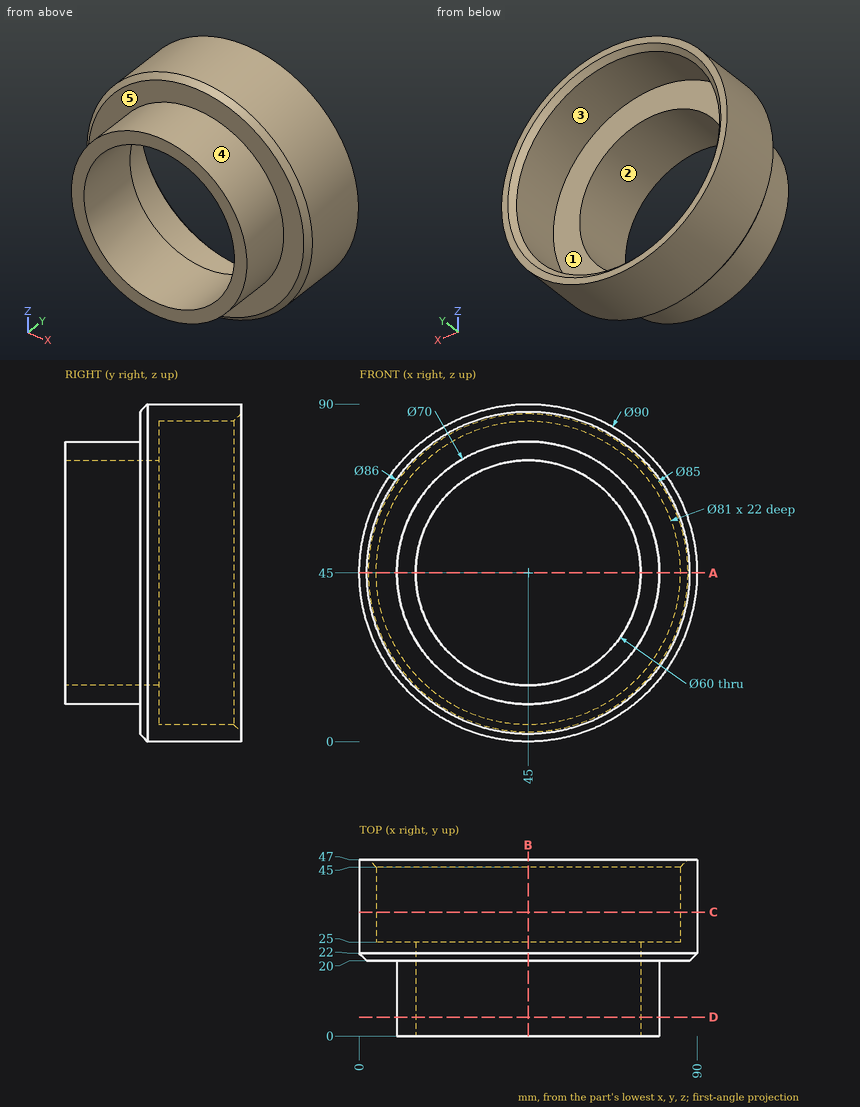
Could you check a few things on this drawing? It's one solid part, dimensions in mm from its lowest x, y, z. A direction names the side the tool comes from. Give positions to 0.01 mm unless a question says otherwise; leave off trailing zeros. Write each loop counter-clockwise with the first axis right and the second up, starting at its lowest first coordinate (ties: lowest second). Pieces come first, ordered by that corner, then holes.
(1) Imagine slicing it at A-A, the plane z = 45. Write out the boundary of the cut face in (x, y), and give its area (3 significant figures).
Output values:
outline: (0, 22) - (2, 20) - (10, 20) - (10, 0) - (15, 0) - (15, 25) - (4.5, 25) - (4.5, 45) - (2.5, 47) - (0, 47) - close; (75, 0) - (80, 0) - (80, 20) - (88, 20) - (90, 22) - (90, 47) - (87.5, 47) - (85.5, 45) - (85.5, 25) - (75, 25) - close
area: 540 mm2
(2) On a 3-axis mill with a long thin cutter (end or side, diameter ignored), from which of +Z, -Z, +X, -X, +Y, -Y can I reach the whole of each face in a straight line? I mean the marked faces 1 and 2. Say none if no direction works.
Output values:
face 1: +Y
face 2: +Y, -Y
(3) Imagine slicing it at D-D, the plane y = 5. Write out the boundary of the cut face in (x, z), and give its area (3 significant figures).
Output values:
outline: circle Ø70 at (45, 45); hole circle Ø60 at (45, 45)
area: 1,020 mm2
(4) If I drill on L1, parallel to X at y = 15.5, z = 45; L2, parallel to X at y = 35, z = 45, over which ranges is the centre line in solid material (lowest first)?
Output values:
L1: x = 10 to 15, 75 to 80
L2: x = 0 to 4.5, 85.5 to 90
(5) Will these pins go through, and if not, where does the flat tip stop? pin 1 (8 mm diameter, centred on y = 33.5, z = 65.5, fed in from -X); pin 2 (6 mm diameter, centred on x = 69.5, z = 26.5, fed in from +Y); pin 3 (1 mm diameter, centred on y = 5.5, z = 61, fed in from -X).
Output values:
pin 1: stops at x = 3.13
pin 2: stops at y = 25
pin 3: stops at x = 13.62
(6) Thinking about a two-plate mould opening in X: for the marked faces 3, 4 and 5, which applies, pulls with the +X half, pulls with the -X half, needs draft (parallel to the pull), parting line crosses it, or undercut?
Output values:
face 3: undercut
face 4: parting line crosses it
face 5: needs draft
(7) Imagine slicing it at B-B, the plane x = 45. Write out the boundary of the cut face in (y, z), and give its area (3 significant figures).
Output values:
outline: (0, 10) - (20, 10) - (20, 2) - (22, 0) - (47, 0) - (47, 2.5) - (45, 4.5) - (25, 4.5) - (25, 15) - (0, 15) - close; (0, 75) - (25, 75) - (25, 85.5) - (45, 85.5) - (47, 87.5) - (47, 90) - (22, 90) - (20, 88) - (20, 80) - (0, 80) - close
area: 540 mm2
(8) Imagine slicing it at C-C, the plane y = 33. Write out the boundary of the cut face in (x, z).
Output values:
outline: circle Ø90 at (45, 45); hole circle Ø81 at (45, 45)
